Can you work these out from the model? Positions are in its coordinate system, mm. A direction names the side the tool comes from. Coordinates: 2 decimals unless noted, no trailing zeros. Loops run counter-clockwise (first coordinate to the right, second up) from the corner with the lowest first, then second, coordinate; pieces in that order, holes last. Notation, with made-up numbers: M 66.25,67 L 78.25,67 A20 cw 78.25,94 Z; hole C -36,-19.75 d3. An arc over 180 degrees is marked long. Return JSON: item names as keys, results as strings. Group by question number.
```python
from build123d import *

# Parameters (mm, degrees)
SKETCH_1_R      = 140
SKETCH_1_R_2    = 47.5
SKETCH_1_R_3    = 10
EXTRUDE_1_DEPTH = 10
SKETCH_2_R      = 100
SKETCH_2_R_2    = 90
EXTRUDE_2_DEPTH = 32.5


with BuildPart() as part:
    # 草图1 → 拉伸1 (new body)
    with BuildSketch(Plane.XY):
        Circle(SKETCH_1_R)
        Circle(SKETCH_1_R_2, mode=Mode.SUBTRACT)
        with Locations((0, 120)):
            Circle(SKETCH_1_R_3, mode=Mode.SUBTRACT)
        with Locations((120, 0)):
            Circle(SKETCH_1_R_3, mode=Mode.SUBTRACT)
        with Locations((0, -120)):
            Circle(SKETCH_1_R_3, mode=Mode.SUBTRACT)
        with Locations((-120, 0)):
            Circle(SKETCH_1_R_3, mode=Mode.SUBTRACT)
    extrude(amount=EXTRUDE_1_DEPTH)

    # 草图2 → 拉伸2 (add)
    with BuildSketch(Plane.XY.offset(10)):
        Circle(SKETCH_2_R)
        Circle(SKETCH_2_R_2, mode=Mode.SUBTRACT)
    extrude(amount=EXTRUDE_2_DEPTH)


solid = part.part
```
1) Suppose I cut it at C-C, the plane y = -38. List the corners of the cut face in (x, z) for me.
2) Suppose I cut it at A-A, the plane y = 0. List the corners of the cut face in (x, z) for me, then the cut area to 3 significant figures.
3) For pin 1 (12 mm diameter, centred on y = 60.5, z = 21, fed in from -X); pin 2 (23 mm diameter, centred on x = 0, y = -120, fed in from +Z); pin 3 (12 mm diameter, centred on y = 93, z = 15, fed in from -X); pin 4 (12 mm diameter, centred on x = 120, y = 0, fed in from +Z), each with a flat end and sliding along its axis, tell me the tip position at first contact or that it passes through.
4) If we mould it in two halves opening along Y, with no side actions, what happens to faces 1 (the face through (93, 42, 10)), 2 (the face through (110, 0, 5)), 3 (the face through (95.38, 30.04, 26.02))? For each: +Y half, -Y half, draft (parallel to the pull), parting line (faces both ways), or undercut.
5) For faces 4 (the face through (39, -39, 10)), 5 (the face through (5.38, 128.43, 4.93)), which set-ups out of +Z, -Z, +X, -X, +Y, -Y let a thin tool reach every point of the face, with its end or its side?
6) If I drill on line 1 (Y direction, x = 0, z = 7); line 2 (Y direction, x = 0, z = 17); line 3 (X direction, y = -13, z = 15), over which ranges is the centre line in solid material (lowest first)? Write a range as from..to.
7) Suppose I cut it at D-D, the plane x = 120. List the corners of the cut face in (y, z) for me.
Returned:
{
 "1": {"outline": "M -134.74,0 L -28.5,0 L -28.5,10 L -81.58,10 L -81.58,42.5 L -92.5,42.5 L -92.5,10 L -134.74,10 Z; M 28.5,0 L 134.74,0 L 134.74,10 L 92.5,10 L 92.5,42.5 L 81.58,42.5 L 81.58,10 L 28.5,10 Z"},
 "2": {"outline": "M -140,0 L -130,0 L -130,10 L -140,10 Z; M -110,0 L -47.5,0 L -47.5,10 L -90,10 L -90,42.5 L -100,42.5 L -100,10 L -110,10 Z; M 47.5,0 L 110,0 L 110,10 L 100,10 L 100,42.5 L 90,42.5 L 90,10 L 47.5,10 Z; M 130,0 L 140,0 L 140,10 L 130,10 Z", "area": "2,100 mm²"},
 "3": {"pin 1": "stops at x = -83.84", "pin 2": "stops at z = 10", "pin 3": "stops at x = -107.5", "pin 4": "passes through"},
 "4": {"face 1": "draft", "face 2": "undercut", "face 3": "parting line"},
 "5": {"face 4": "+Z", "face 5": "+Z, -Z"},
 "6": {"line 1": "y = -140..-130, -110..-47.5, 47.5..110, 130..140", "line 2": "y = -100..-90, 90..100", "line 3": "x = -99.15..-89.06, 89.06..99.15"},
 "7": {"outline": "M -72.11,0 L -10,0 L -10,10 L -72.11,10 Z; M 10,0 L 72.11,0 L 72.11,10 L 10,10 Z"}
}
